```python
from build123d import *

# Parameters (mm, degrees)
MODEL_R             = 3.781579339
MODEL_R_2           = 1.7
MODEL_R_3           = 1.6
MODEL_W             = 12
MODEL_H             = 28
BOSS_EXTRUDE2_DEPTH = 3
SKETCH1_R           = 1.0005
CUT_EXTRUDE1_DEPTH  = 312.964229084


with BuildPart() as part:
    # Model → Boss-Extrude2 (new body)
    with BuildSketch(Plane.XY):
        with BuildLine():
            Line((88, 60), (220, 60))
            Line((220, 60), (254.882583618, 93.640518188))
            Line((254.882583618, 93.640518188), (259.489592216, 106.576108559))
            ThreePointArc((259.489592216, 106.576108559), (259.424141413, 121.57623231), (248.498382723, 131.854159795))
            Line((248.498382723, 131.854159795), (161.617078665, 168.980084934))
            ThreePointArc((161.617078665, 168.980084934), (154.617078665, 170.855729281), (147.617078665, 168.980084934))
            Line((147.617078665, 168.980084934), (59.501617277, 131.854159795))
            ThreePointArc((59.501617277, 131.854159795), (48.575858587, 121.57623231), (48.510407784, 106.576108559))
            Line((48.510407784, 106.576108559), (52.677086204, 96.362955936))
            Line((52.677086204, 96.362955936), (88, 60))
        make_face()
        with Locations((154.617078665, 157.237991333)):
            Circle(MODEL_R, mode=Mode.SUBTRACT)
        with Locations((163.114624023, 157.237991333)):
            Circle(MODEL_R_2, mode=Mode.SUBTRACT)
        with Locations((146.117078665, 157.237991333)):
            Circle(MODEL_R_2, mode=Mode.SUBTRACT)
        with Locations((115.877120948, 132.296819167)):
            Circle(MODEL_R_3, mode=Mode.SUBTRACT)
        with Locations((137.734977924, 66.871509225)):
            Circle(MODEL_R_3, mode=Mode.SUBTRACT)
        with Locations((193.918561918, 129.673741782)):
            Circle(MODEL_R_3, mode=Mode.SUBTRACT)
        with Locations((172.735008, 66.871509225)):
            Circle(MODEL_R_3, mode=Mode.SUBTRACT)
        with Locations((95.2, 104.75)):
            Circle(MODEL_R_3, mode=Mode.SUBTRACT)
        with Locations((85.560630532, 114.806524888)):
            Circle(MODEL_R_3, mode=Mode.SUBTRACT)
        with Locations((224.233700932, 112.158328537)):
            Circle(MODEL_R_2, mode=Mode.SUBTRACT)
        with Locations((95.2, 67.75)):
            Circle(MODEL_R_3, mode=Mode.SUBTRACT)
        with Locations((93, 86)):
            Rectangle(MODEL_W, MODEL_H, mode=Mode.SUBTRACT)
        Polygon((181.734462562, 65.257395619), (181.735489, 68.457395619), (202.735488, 68.450659619), (202.734461562, 65.250659619), align=None, mode=Mode.SUBTRACT)
        Polygon((249.399348556, 95.770313962), (231.216181373, 106.276143646), (232.817069658, 109.046911896), (251.000236841, 98.541082213), align=None, mode=Mode.SUBTRACT)
        Polygon((60.374623433, 98.42894725), (58.775510803, 101.200740676), (76.965405371, 111.694917426), (78.564518, 108.923124), align=None, mode=Mode.SUBTRACT)
        Polygon((128.734464562, 65.274396), (128.735491, 68.474396), (107.735493, 68.481132), (107.734466562, 65.281132), align=None, mode=Mode.SUBTRACT)
        Polygon((142.66224045, 145.902603249), (124.4723462, 135.408426681), (122.873233571, 138.180220108), (136.035908619, 145.774076024), (141.063127638, 148.674396991), align=None, mode=Mode.SUBTRACT)
        Polygon((167.142166, 143.296685), (168.743054285, 146.067453251), (186.926220285, 135.561624251), (185.325332, 132.790856), align=None, mode=Mode.SUBTRACT)
    extrude(amount=BOSS_EXTRUDE2_DEPTH)

    # Sketch1 → Cut-Extrude1 (cut, through all)
    with BuildSketch(Plane.XY.offset(3)):
        with Locations((61.241241971, 98.928919808)):
            Circle(SKETCH1_R)
        with Locations((59.642129342, 101.700713234)):
            Circle(SKETCH1_R)
        with Locations((76.098786832, 111.194944868)):
            Circle(SKETCH1_R)
        with Locations((77.697899462, 108.423151442)):
            Circle(SKETCH1_R)
        with Locations((87.707460335, 99.292539665)):
            Circle(SKETCH1_R)
        with Locations((98.292539665, 99.292539665)):
            Circle(SKETCH1_R)
        with Locations((87.707460335, 72.707460335)):
            Circle(SKETCH1_R)
        with Locations((98.292539665, 72.707460335)):
            Circle(SKETCH1_R)
        with Locations((108.735992948, 68.480811078)):
            Circle(SKETCH1_R)
        with Locations((108.73496651, 65.280811078)):
            Circle(SKETCH1_R)
        with Locations((127.733964613, 65.274716923)):
            Circle(SKETCH1_R)
        with Locations((127.734991051, 68.474716923)):
            Circle(SKETCH1_R)
        with Locations((182.73496251, 65.257074697)):
            Circle(SKETCH1_R)
        with Locations((182.735988949, 68.457074697)):
            Circle(SKETCH1_R)
        with Locations((201.734988051, 68.450980541)):
            Circle(SKETCH1_R)
        with Locations((201.733961613, 65.250980541)):
            Circle(SKETCH1_R)
        with Locations((232.082479384, 105.775615918)):
            Circle(SKETCH1_R)
        with Locations((233.683367669, 108.546384168)):
            Circle(SKETCH1_R)
        with Locations((250.13393883, 99.041609941)):
            Circle(SKETCH1_R)
        with Locations((248.533050545, 96.27084169)):
            Circle(SKETCH1_R)
        with Locations((168.008464011, 142.796157272)):
            Circle(SKETCH1_R)
        with Locations((169.609352296, 145.566925523)):
            Circle(SKETCH1_R)
        with Locations((184.459033989, 133.291383728)):
            Circle(SKETCH1_R)
        with Locations((186.059922274, 136.062151978)):
            Circle(SKETCH1_R)
        with Locations((141.795621912, 145.402630691)):
            Circle(SKETCH1_R)
        with Locations((140.196509099, 148.174424012)):
            Circle(SKETCH1_R)
        with Locations((123.739852109, 138.680192666)):
            Circle(SKETCH1_R)
        with Locations((125.338964739, 135.90839924)):
            Circle(SKETCH1_R)
    extrude(amount=-CUT_EXTRUDE1_DEPTH, mode=Mode.SUBTRACT)


solid = part.part
```
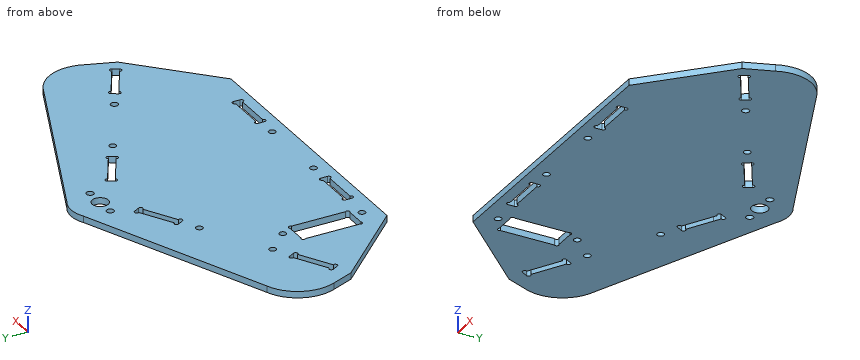
Check sheet for the modelled part. Datum: model origin and axes. Units: mm. Coordinates: 2 decimals unless noted, no trailing zeros. Loops run counter-clockwise (first coordinate to the right, second up) from the corner with the lowest first, then second, coordinate; pieces in that order, holes last.
1) Sectioned sample at B-B (y = 91). Record the boundary of the cut face in (x, z).
2) Sectioned sample at D-D (y = 124). Record the boundary of the cut face in (x, z).
3) Sectioned sample at C-C (z = 0.9). Count the separate pieces of the cut face and the enclosed holes in it, and give its area (3 significant figures).
4) Gauge pin test, flat ends, axial feed: pin 1 (2.5 mm diameter, centred on x = 146.12, y = 157.24, fed in from +Z); pin 2 (0.9 mm diameter, centred on x = 94.5, z = 1, fed in from +Y); pin 3 (0.9 mm diameter, centred on y = 66.5, z = 1, fed in from -X); pin 4 (0.9 mm diameter, centred on y = 87, z = 1.5, fed in from -X). Record the tip position at first contact, or that the pin passes through.
5) Material ranges on probe 1 along X at (y, z) = (157, 2.65); probe 2 along Y at (x, z) = (95.2, 0.8); probe 3 along Y at (x, z) = (95, 0.45), recorded low to high.
6) Sectioned sample at A-A (x = 66). Record the boundary of the cut face in (y, z), and give its area (3 significant figures).
Check sheet entries:
1. outline: (57.89, 0) - (87, 0) - (87, 3) - (57.89, 3) - close; (99, 0) - (252.14, 0) - (252.14, 3) - (99, 3) - close
2. outline: (49.84, 0) - (258.16, 0) - (258.16, 3) - (49.84, 3) - close
3. separate pieces: 1
3. enclosed holes: 18
3. area: 16,400 mm2
4. pin 1: passes through
4. pin 2: stops at y = 146.79
4. pin 3: stops at x = 81.25
4. pin 4: stops at x = 61.34
5. probe 1: x = 119.18 to 144.43, 147.8 to 150.84, 158.39 to 161.43, 164.8 to 189.65
5. probe 2: y = 60 to 66.15, 69.35 to 72, 100 to 103.15, 106.35 to 146.9
5. probe 3: y = 60 to 66.16, 69.34 to 72, 100 to 103.16, 106.34 to 146.81
6. outline: (82.65, 0) - (101.67, 0) - (101.67, 3) - (82.65, 3) - close; (105.37, 0) - (134.59, 0) - (134.59, 3) - (105.37, 3) - close
6. area: 145 mm2
